CAD build for the part. Positions are in the model's coordinates, mm. A direction names the side the tool comes from. Give positions to 0.01 mm unless a question says otherwise; leave off trailing zeros. Order: outer loops, then holes, each group sorted by start corner. A loop starts at its lowest first (then second) coordinate and runs counter-clockwise, first axis right, second up. Notation, with made-up numbers: M -30.75,22.5 L 19.25,22.5 A13 ccw 19.25,35.5 Z; hole C -24.75,25.5 d7. An arc over 180 degrees is marked long. Put each result on its own line as item: value. Start each with the question number.
1) Cut at A-A (x = 0). Write the cut outline in (y, z), and give its area (3 significant figures).
2) Two-plate mould, pull along X, no slides. Class faces 3 (the face through (-9.538, 60.146, 42.954)), 4 (the face through (-36, 122, -23)), 5 (the face through (-37, 22, -16)): released by +X, released by -X, zero draft, split by the parting line, or undercut.
3) Drill centre lines: line 1 (X direction, y = 58, z = 0); line 2 (Z direction, x = 0, y = 17). Where is each one in solid material? Low to high. Write a range as [from, to].
4) Pin check, flat tips, straight feed: pin 1 (1 mm diameter, centred on y = 93, z = 9, fed in from +X); pin 2 (6 mm diameter, centred on y = 53, z = 22.5, fed in from -X); pin 3 (8 mm diameter, centred on y = 61, z = 18.5, fed in from -X). Stop position of each tip, or through.
5) Cut at B-B (z = 0). Write the cut outline in (x, y).
6) Tool access for faces 1 (the face through (-8.67, 10.85, 39.05)), 2 (the face through (-33.727, 131.86, 25.861)): list every direction of +Z, -Z, +X, -X, +Y, -Y with a clear straight run to the whole face (end or side of a thin tool).
7) Cut at C-C (y = 99). Write the cut outline in (x, z).
```python
from build123d import *

# Parameters (mm, degrees)
SKETCH1_R           = 44
SKETCH1_R_2         = 40
BOSS_EXTRUDE1_DEPTH = 22
SKETCH2_R           = 44
SKETCH2_R_2         = 41.68814
BOSS_EXTRUDE2_DEPTH = 100
SKETCH3_R           = 42.5
SKETCH3_R_2         = 41.68814
BOSS_EXTRUDE3_DEPTH = 20


with BuildPart() as part:
    # Sketch1 → Boss-Extrude1 (new body)
    with BuildSketch(Plane(origin=(0, 0, 0), x_dir=(1, 0, 0), z_dir=(0, 1, 0))):
        Circle(SKETCH1_R)
        Circle(SKETCH1_R_2, mode=Mode.SUBTRACT)
    extrude(amount=BOSS_EXTRUDE1_DEPTH)

    # Sketch2 → Boss-Extrude2 (add)
    with BuildSketch(Plane(origin=(0, 22, 0), x_dir=(1, 0, 0), z_dir=(0, 1, 0))):
        Circle(SKETCH2_R)
        Circle(SKETCH2_R_2, mode=Mode.SUBTRACT)
    extrude(amount=BOSS_EXTRUDE2_DEPTH)

    # Sketch3 → Boss-Extrude3 (add)
    with BuildSketch(Plane(origin=(0, 122, 0), x_dir=(1, 0, 0), z_dir=(0, 1, 0))):
        Circle(SKETCH3_R)
        Circle(SKETCH3_R_2, mode=Mode.SUBTRACT)
    extrude(amount=BOSS_EXTRUDE3_DEPTH)


solid = part.part
```
Solution:
1. outline: M 0,-44 L 122,-44 L 122,-42.5 L 142,-42.5 L 142,-41.69 L 22,-41.69 L 22,-40 L 0,-40 Z; M 0,40 L 22,40 L 22,41.69 L 142,41.69 L 142,42.5 L 122,42.5 L 122,44 L 0,44 Z
1. area: 671 mm²
2. face 3: split by the parting line
2. face 4: zero draft
2. face 5: undercut
3. line 1: [-44, -41.69], [41.69, 44]
3. line 2: [-44, -40], [40, 44]
4. pin 1: x = 43.17
4. pin 2: x = -39.44
4. pin 3: x = -41.54
5. outline: M -44,0 L -40,0 L -40,22 L -41.69,22 L -41.69,142 L -42.5,142 L -42.5,122 L -44,122 Z; M 40,0 L 44,0 L 44,122 L 42.5,122 L 42.5,142 L 41.69,142 L 41.69,22 L 40,22 Z
6. face 1: +Y, -Y
6. face 2: +Y
7. outline: C 0,0 d88; hole C 0,0 d83.38
